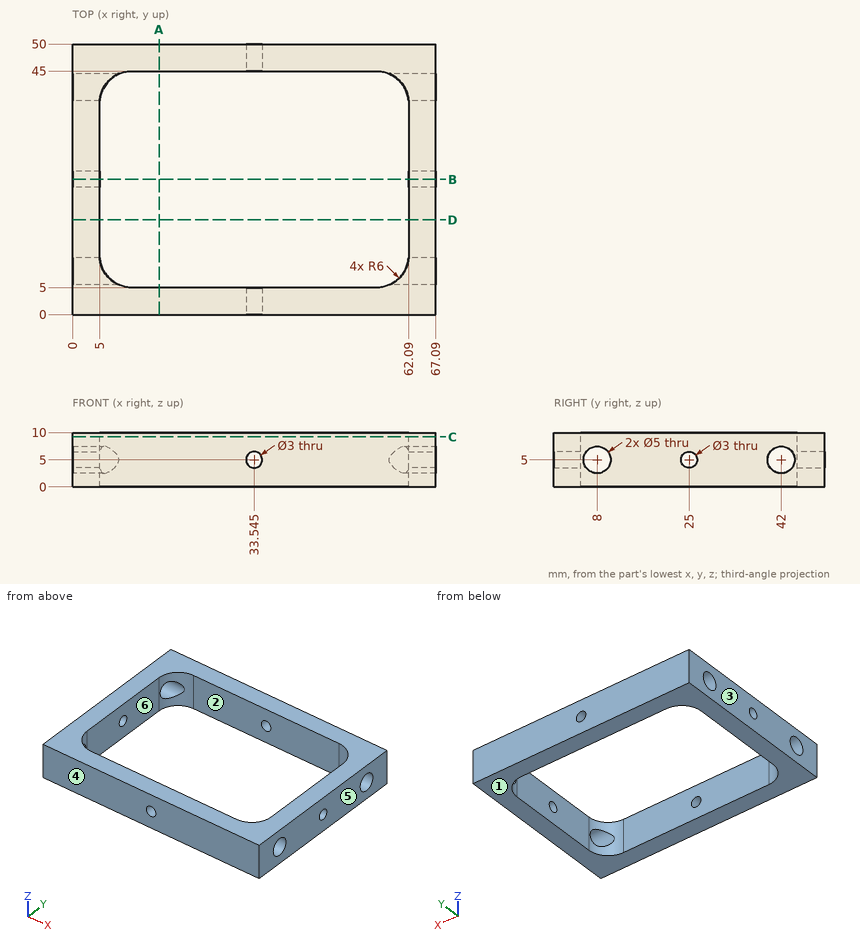
Answer from the drawing. Dimensions are ordinates in mm from the lowest x, y and z of the part. A direction names the side the tool comes from. Coordinates: 2 decimals unless noted, no trailing zeros. Order: outer loops, then holes, each group sorted by start corner. A loop starts at its lowest first (then second) coordinate and runs counter-clockwise, first axis right, second up. Notation, with made-up numbers: M -1,19.5 L 53,19.5 A21 ccw 53,57.5 Z; hole C -31.5,0 d4. An arc over 180 degrees is marked long. Put each result on its own line as item: value. Start each with the question number.
Item 1: Consider probe 1 along Y at (x, z) = (63.75, 5); probe 2 along Y at (x, z) = (56.5, 2.75); probe 3 along X at (y, z) = (26.5, 1.75). Determine where each line is inside the solid, lowest interval first. Write a range as [from, to].
Item 2: Given pin 1 Ø3.5 at (y, z) = (25, 5) entering from +X; pin 2 Ø2.5 at (x, z) = (33.545, 5) entering from +Y, each flat-ended and moving along its own axis, determine where each tip first touches the part or whether it passes through.
Item 3: Section A-A, the plane x = 16 is taken. Determine the outline of the cut face in (y, z).
Item 4: The mould has two halves that part along X. Classify the marked faces 3, 4, 5 and 6: +X half, -X half, draft (parallel to the pull), parting line (faces both ways), or undercut.
Item 5: Section B-B, the plane y = 25 is taken. Determine the outline of the cut face in (x, z).
Item 6: Section C-C, the plane z = 9.25 is taken. Determine the outline of the cut face in (x, y).
Item 7: For the marked faces 1 and 2, determine the directions among +Z, -Z, +X, -X, +Y, -Y from which every point of the face is accessible in a straight line to the end or side of a thin tool.
Item 8: Section D-D, the plane y = 17.5 is taken. Determine the outline of the cut face in (x, z).
Computed:
1. probe 1: y = [0, 5.5], [10.5, 23.5], [26.5, 39.5], [44.5, 50]
1. probe 2: y = [0, 5.01], [44.99, 50]
1. probe 3: x = [0, 5], [62.09, 67.09]
2. pin 1: stops at x = 67.09
2. pin 2: passes through
3. outline: M 0,0 L 5,0 L 5,10 L 0,10 Z; M 45,0 L 50,0 L 50,10 L 45,10 Z
4. face 3: -X half
4. face 4: draft
4. face 5: +X half
4. face 6: undercut
5. outline: M 0,0 L 5,0 L 5,3.5 L 0,3.5 Z; M 0,6.5 L 5,6.5 L 5,10 L 0,10 Z; M 62.09,0 L 67.09,0 L 67.09,3.5 L 62.09,3.5 Z; M 62.09,6.5 L 67.09,6.5 L 67.09,10 L 62.09,10 Z
6. outline: M 0,0 L 67.09,0 L 67.09,50 L 0,50 Z; hole M 5,11 A6 ccw 11,5 L 56.09,5 A6 ccw 62.09,11 L 62.09,39 A6 ccw 56.09,45 L 11,45 A6 ccw 5,39 Z
7. face 1: -Z, +X, -X, +Y, -Y
7. face 2: +Z, -Z
8. outline: M 0,0 L 5,0 L 5,10 L 0,10 Z; M 62.09,0 L 67.09,0 L 67.09,10 L 62.09,10 Z
